Work out the finished part from the listing and answer in its coordinate system (mm). A direction names the side the tool comes from. Coordinates: 2 decimals unless noted, no trailing zeros. Loops run counter-clockwise (first coordinate to the right, second up) from the corner with the lowest first, then second, coordinate; pieces in that order, holes last. Notation, with made-up numbers: (64.5, 75.5) -> (89.5, 75.5) arc R34 ccw to (89.5, 106.5) -> close; hole circle Ø8 at (18.25, -1). An arc over 180 degrees is marked (long way). Use a Markdown table: item, result.
from build123d import *

# Parameters (mm, degrees)
EXTRUDE_1_DEPTH     = 30
SKETCH_2_R          = 7.5
EXTRUDE_2_DEPTH     = 20
SKETCH_3_W          = 55
SKETCH_3_H          = 30
EXTRUDE_3_DEPTH     = 20
SKETCH_4_R          = 5
CUT_EXTRUDE_1_DEPTH = 10


with BuildPart() as part:
    # 草图1 → 凸台-拉伸1 (new body)
    with BuildSketch(Plane.XY):
        Polygon((-52.460777496, 0), (197.539222504, 0), (172.539222504, 43.301270189), (-27.460777496, 43.301270189), align=None)
    extrude(amount=EXTRUDE_1_DEPTH)

    # 草图2 → 凸台-拉伸2 (add)
    with BuildSketch(Plane(origin=(0, 0, 0), x_dir=(-1, 0, 0), z_dir=(0, 0, -1))):
        with Locations(Location((-72.539222504, 20.626682139, 0), (0, 0, 180))):
            Circle(SKETCH_2_R)
    extrude(amount=EXTRUDE_2_DEPTH)

    # 草图3 → 凸台-拉伸3 (add)
    with BuildSketch(Plane(origin=(0, 0, -20), x_dir=(-1, 0, 0), z_dir=(0, 0, -1))):
        with Locations((-72.539222504, 20.626682139)):
            Rectangle(SKETCH_3_W, SKETCH_3_H)
    extrude(amount=EXTRUDE_3_DEPTH)

    # 草图4 → 切除-拉伸1 (cut)
    with BuildSketch(Plane(origin=(0, 0, -40), x_dir=(-1, 0, 0), z_dir=(0, 0, -1))):
        with Locations((-72.539222504, 20.626682139)):
            Circle(SKETCH_4_R)
    extrude(amount=-CUT_EXTRUDE_1_DEPTH, mode=Mode.SUBTRACT)


solid = part.part
Q1. Section C-C on x = 160 is taken. Determine the outline of the cut face in (y, z).
Solved:
| item | result |
|---|---|
| outline | (0, 0) -> (43.3, 0) -> (43.3, 30) -> (0, 30) -> close |
Q2. Section B-B on z = -23.5 is taken. Determine the outline of the cut face in (x, y), and give its area (3 significant figures).
Solved:
| item | result |
|---|---|
| outline | (45.04, 5.63) -> (100.04, 5.63) -> (100.04, 35.63) -> (45.04, 35.63) -> close |
| area | 1,650 mm² |
Q3. Given pin 1 Ø10 at (y, z) = (5, -25.5) entering from -X; pin 2 Ø6 at (y, z) = (22.5, -26) entering from +X; pin 3 Ø8 at (x, z) = (81, -15.5) entering from -Y, each flat-ended and moving along its own axis, determine where each tip first touches the part or whether it passes through.
Solved:
| item | result |
|---|---|
| pin 1 | x = 45.04 |
| pin 2 | x = 100.04 |
| pin 3 | y = 14.6 |
Q4. Section A-A on y = 8 is taken. Determine the outline of the cut face in (x, z), and give its area (3 significant figures).
Solved:
| item | result |
|---|---|
| outline | (-47.84, 0) -> (192.92, 0) -> (192.92, 30) -> (-47.84, 30) -> close; (45.04, -40) -> (100.04, -40) -> (100.04, -20) -> (45.04, -20) -> close |
| area | 8,320 mm² |
Q5. Section D-D on y = 31 is taken. Determine the outline of the cut face in (x, z), and give its area (3 significant figures).
Solved:
| item | result |
|---|---|
| outline | (-34.56, 0) -> (179.64, 0) -> (179.64, 30) -> (-34.56, 30) -> close; (45.04, -40) -> (100.04, -40) -> (100.04, -20) -> (45.04, -20) -> close |
| area | 7,530 mm² |
Q6. Determine the mould class of faces 1 (the flat face through (71, 22, 30)), 2 (the flat face through (73, 5.627, -30)), 3 (the flat face through (67, 28, -20)) for opening direction Z: pulls with the +Z half, pulls with the -Z half, needs draft (parallel to the pull), parting line crosses it, or undercut.
Solved:
| item | result |
|---|---|
| face 1 | pulls with the +Z half |
| face 2 | needs draft |
| face 3 | undercut |
Q7. For faces 4 (the flat face through (73, 35.627, -30)), 5 (the flat face through (100.039, 20, -30)), 6 (the cylindrical face through (79.7, 18.4, -9.9)), 7 (the flat face through (45.039, 20, -30)), 8 (the cylindrical face through (67.92, 18.71, -35.07)), determine the directions among +Z, -Z, +X, -X, +Y, -Y from which every point of the face is accessible in a straight line to the end or side of a thin tool.
Solved:
| item | result |
|---|---|
| face 4 | -Z, +X, -X, +Y |
| face 5 | -Z, +X, +Y, -Y |
| face 6 | none |
| face 7 | -Z, -X, +Y, -Y |
| face 8 | -Z |
Q8. Consider line 1 (Z direction, x = 91, y = 34.5); line 2 (Z direction, x = 5, y = 38); line 3 (X direction, y = 22.5, z = -28). Determine where each line is inside the solid, lowest interval first. Write a range as [from, to].
Solved:
| item | result |
|---|---|
| line 1 | [-40, -20], [0, 30] |
| line 2 | [0, 30] |
| line 3 | [45.04, 100.04] |
